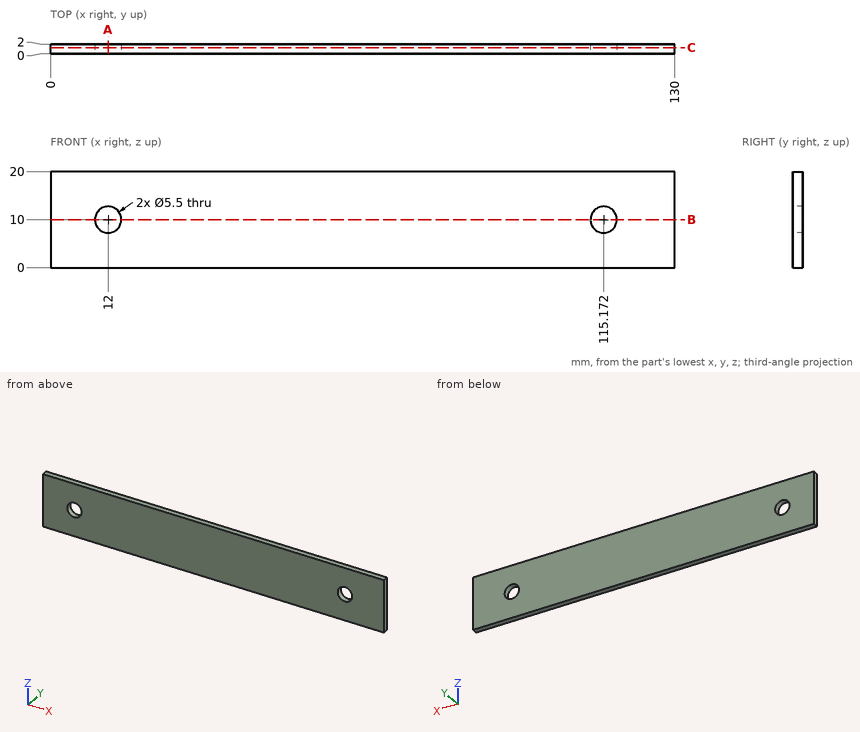
Print and shaded views of the part. All mm, measured from the part's lowest x, y and z. Coordinates: 2 decimals unless noted, no trailing zeros. Write each loop counter-clockwise with the first axis right and the second up, starting at its lowest first coordinate (ties: lowest second). Pieces come first, ordered by that corner, then holes.
(1) Cut at B-B, the plane z = 10. List the corners of the cut face in (x, y).
(2) Cut at C-C, the plane y = 1.25. List the corners of the cut face in (x, z).
(3) Drill centre lines: probe 1 along X at (y, z) = (0.45, 10); probe 2 along Z at (x, y) = (12, 1.4); probe 3 along X at (y, z) = (1.35, 12.5). Where is each one in solid material? Low to high.
(4) Cut at A-A, the plane x = 12. List the corners of the cut face in (y, z), and give its area (3 significant figures).
(5) Flat gauge pins, fed straight in: pin 1 (2 mm diameter, centred on x = 96, z = 8, fed in from -Y); pin 2 (3.5 mm diameter, centred on x = 115.172, z = 10, fed in from -Y). Where does each tip first touch, or does it go through?
Geometry says:
1. outline: (0, 0) - (9.25, 0) - (9.25, 2) - (0, 2) - close; (14.75, 0) - (112.42, 0) - (112.42, 2) - (14.75, 2) - close; (117.92, 0) - (130, 0) - (130, 2) - (117.92, 2) - close
2. outline: (0, 0) - (130, 0) - (130, 20) - (0, 20) - close; hole circle Ø5.5 at (12, 10); hole circle Ø5.5 at (115.17, 10)
3. probe 1: x = 0 to 9.25, 14.75 to 112.42, 117.92 to 130
3. probe 2: z = 0 to 7.25, 12.75 to 20
3. probe 3: x = 0 to 10.85, 13.15 to 114.03, 116.32 to 130
4. outline: (0, 0) - (2, 0) - (2, 7.25) - (0, 7.25) - close; (0, 12.75) - (2, 12.75) - (2, 20) - (0, 20) - close
4. area: 29.0 mm2
5. pin 1: stops at y = 0
5. pin 2: passes through
